Can you work these out from the model? Positions are in its coordinate system, mm. A direction names the side the tool comes from. Give positions to 0.01 mm unless a question says otherwise; leave off trailing zeros. Order: outer loops, then holes, each group sorted by start corner. A loop starts at its lowest first (then second) coordinate and runs counter-clockwise, first axis right, second up. Notation, with made-up numbers: M 18,19.5 L 32,19.5 A30 cw 32,42.5 Z; hole C -34,-37.75 d5. An arc over 180 degrees is marked long. Answer as a JSON object with one key per item and string values.
```python
from build123d import *

# Parameters (mm, degrees)
SKETCH_1_W          = 20
SKETCH_1_H          = 20
EXTRUDE_1_DEPTH     = 500
SKETCH_2_W          = 20
SKETCH_2_H          = 10
CUT_EXTRUDE_1_DEPTH = 10.5
SKETCH_3_R          = 4
CUT_EXTRUDE_2_DEPTH = 21
SKETCH_4_W          = 20.5
SKETCH_4_H          = 10
CUT_EXTRUDE_5_DEPTH = 21
SKETCH_5_R          = 4
CUT_EXTRUDE_4_DEPTH = 21
SKETCH_6_R          = 4
CUT_EXTRUDE_6_DEPTH = 501.49975025
SKETCH_7_W          = 17
SKETCH_7_H          = 17
CUT_EXTRUDE_7_DEPTH = 501.199960016


with BuildPart() as part:
    # ｽｹｯﾁ1 → ﾎﾞｽ - 押し出し1 (new body)
    with BuildSketch(Plane.XY):
        Rectangle(SKETCH_1_W, SKETCH_1_H)
    extrude(amount=EXTRUDE_1_DEPTH)

    # ｽｹｯﾁ2 → ｶｯﾄ - 押し出し1 (cut, symmetric)
    with BuildSketch(Plane.XY.offset(325)):
        with Locations((0, 5)):
            Rectangle(SKETCH_2_W, SKETCH_2_H)
    cut_extrude_1 = extrude(amount=CUT_EXTRUDE_1_DEPTH, both=True, mode=Mode.SUBTRACT)

    # ﾐﾗｰ1: ｶｯﾄ - 押し出し1 across plane
    add(cut_extrude_1.mirror(Plane.XY.offset(250)), mode=Mode.SUBTRACT)

    # ｽｹｯﾁ3 → ｶｯﾄ - 押し出し2 (cut)
    with BuildSketch(Plane.XZ.offset(10)):
        with Locations(Location((0, 325, 0), (0, 0, 270))):
            Circle(SKETCH_3_R)
        with Locations(Location((0, 175, 0), (0, 0, 270))):
            Circle(SKETCH_3_R)
    extrude(amount=-CUT_EXTRUDE_2_DEPTH, mode=Mode.SUBTRACT)

    # ｽｹｯﾁ4 → ｶｯﾄ - 押し出し5 (cut)
    with BuildSketch(Plane(origin=(10, 0, 0), x_dir=(0, 0, -1), z_dir=(1, 0, 0))):
        with Locations((-10.25, -5)):
            Rectangle(SKETCH_4_W, SKETCH_4_H)
    cut_extrude_5 = extrude(amount=-CUT_EXTRUDE_5_DEPTH, mode=Mode.SUBTRACT)

    # ｽｹｯﾁ5 → ｶｯﾄ - 押し出し4 (cut)
    with BuildSketch(Plane.XZ.offset(10)):
        with Locations(Location((0, 10, 0), (0, 0, 270))):
            Circle(SKETCH_5_R)
        with Locations((0, 510.5)):
            Circle(SKETCH_5_R)
    cut_extrude_4 = extrude(amount=-CUT_EXTRUDE_4_DEPTH, mode=Mode.SUBTRACT)

    # ﾐﾗｰ3: ｶｯﾄ - 押し出し5 across plane
    add(cut_extrude_5.mirror(Plane.XY.offset(250)), mode=Mode.SUBTRACT)

    # ﾐﾗｰ4: ｶｯﾄ - 押し出し4 across plane
    add(cut_extrude_4.mirror(Plane.XY.offset(250)), mode=Mode.SUBTRACT)

    # ｽｹｯﾁ6 → ｶｯﾄ - 押し出し6 (cut, through all)
    with BuildSketch(Plane(origin=(10, 0, 0), x_dir=(0, 0, -1), z_dir=(1, 0, 0))):
        with Locations(Location((-35, 0, 0), (0, 0, 90))):
            Circle(SKETCH_6_R)
        with Locations(Location((-465, 0, 0), (0, 0, 90))):
            Circle(SKETCH_6_R)
    extrude(amount=-CUT_EXTRUDE_6_DEPTH, mode=Mode.SUBTRACT)

    # ｽｹｯﾁ7 → ｶｯﾄ - 押し出し7 (cut, through all)
    with BuildSketch(Plane(origin=(0, 0, 0), x_dir=(-1, 0, 0), z_dir=(0, 0, -1))):
        Rectangle(SKETCH_7_W, SKETCH_7_H)
    extrude(amount=-CUT_EXTRUDE_7_DEPTH, mode=Mode.SUBTRACT)


solid = part.part
```
1) I want a section at A-A on z = 450.5. Write out the boundary of the cut face in (x, y), and give its area (3 significant figures).
Results found:
{"outline": "M -10,-10 L 10,-10 L 10,10 L -10,10 Z; hole M -8.5,-8.5 L 8.5,-8.5 L 8.5,8.5 L -8.5,8.5 Z", "area": "111 mm²"}
2) Thinking about a two-plate mould opening in Y: for faces 1 (the face through (0, 10, 249)), 2 (the face through (-8.5, 0, 246)), 3 (the face through (-10, 0, 246)), which applies, pulls with the +Y half, pulls with the -Y half, needs draft (parallel to the pull), parting line crosses it, or undercut?
Results found:
{"face 1": "pulls with the +Y half", "face 2": "undercut", "face 3": "needs draft"}
3) I'm going to push flat-ended pins straight in: pin 1 Ø5 at (x, y) = (1, 5) entering from -Z (3 decimals); pin 2 Ø5 at (x, y) = (1, -7) entering from +Z; pin 3 Ø1.2 at (x, z) = (9.5, 330) entering from +Y; pin 4 Ø0.8 at (x, z) = (-9, 488) entering from -Y. Where does each tip first touch, or does it pass through?
Results found:
{"pin 1": "passes through", "pin 2": "stops at z = 479.5", "pin 3": "stops at y = 0", "pin 4": "stops at y = 0"}
4) For faces 4 (the face through (0, -9, 329)), 5 (the face through (0, 9, 164.5)), 6 (the face through (0, 8.5, 81)), which set-ups out of +Z, -Z, +X, -X, +Y, -Y let a thin tool reach every point of the face, with its end or its side?
Results found:
{"face 4": "+Y, -Y", "face 5": "+X, -X, +Y", "face 6": "+Z, -Z"}
5) I need wall thicknesses on L1, parallel to Y at x = 3.25, z = 275.5; L2, parallel to Y at x = -8.9, z = 465. Which ranges of each line are inside material? Lowest first, please.
Results found:
{"L1": "y = -10 to -8.5, 8.5 to 10", "L2": "y = -10 to -4, 4 to 10"}
